```python
from build123d import *

# Parameters (mm, degrees)
SKETCH1_W             = 50.8
SKETCH1_H             = 50.8
SKETCH1_R             = 5.55625
BOSS_EXTRUDE1_DEPTH   = 1.5875
F_8_CLEARANCE_HOLE1_D = 4.3053
FILLET1_R             = 2.54


with BuildPart() as part:
    # Sketch1 → Boss-Extrude1 (new, symmetric)
    with BuildSketch(Plane.XY):
        Rectangle(SKETCH1_W, SKETCH1_H)
        Circle(SKETCH1_R, mode=Mode.SUBTRACT)
    extrude(amount=BOSS_EXTRUDE1_DEPTH, both=True)

    # #8 Clearance Hole1 (through all)
    with Locations(Plane.XY.offset(1.5875)):
        with Locations((-15.875, 15.875), (15.875, 15.875), (15.875, -15.875), (-15.875, -15.875), (0, 0)):
            Hole(F_8_CLEARANCE_HOLE1_D / 2)

    # Fillet1
    fillet1_edges = [part.edges().sort_by_distance(p)[0] for p in [
        (25.4, -25.4, 0),
        (-25.4, -25.4, 0),
        (-25.4, 25.4, 0),
        (25.4, 25.4, 0),
    ]]
    fillet(fillet1_edges, radius=FILLET1_R)


solid = part.part
```
Model file for the job. Use its own axes, mm. Coordinates: 2 decimals unless noted, no trailing zeros. Write each loop counter-clockwise with the first axis right and the second up, starting at its lowest first coordinate (ties: lowest second). Pieces come first, ordered by that corner, then holes. Notation, with made-up numbers: (9, 37.5) - (25, 37.5) arc R16 cw to (25, 66.5) - close; hole circle Ø9 at (42.5, 89.5). An arc over 180 degrees is marked (long way). One line per item, written item: value. Start each with the question number.
1. Probe line 1 (Y direction, x = 14, z = 0.15); line 2 (X direction, y = -17.5, z = 0.85); line 3 (Y direction, x = 0, z = -0.55). List the from-to ranges inside material, lowest first. Write a range as from..to.
2. Slice it at B-B (x = 2). Write the cut outline in (y, z), plus the area to 3 significant figures.
3. Mould opens along Y. For faces 1 (the cylindrical face through (-15.59, 18.01, -0.02)), 2 (the flat face through (25.4, 0, 0)), 3 (the flat face through (0, 25.4, 0)) say: released by +Y, released by -Y, zero draft, split by the parting line, or undercut.
4. Slice it at A-A (y = 0). Write the cut outline in (x, z).
5. Slice it at C-C (z = -0.85). Write the cut outline in (x, y) (1 decimal).
Answers below:
1. line 1: y = -25.4..-16.93, -14.82..14.82, 16.93..25.4
1. line 2: x = -25.4..-17.29, -14.46..14.46, 17.29..25.4
1. line 3: y = -25.4..-5.56, 5.56..25.4
2. outline: (-25.4, -1.59) - (-5.18, -1.59) - (-5.18, 1.59) - (-25.4, 1.59) - close; (5.18, -1.59) - (25.4, -1.59) - (25.4, 1.59) - (5.18, 1.59) - close
2. area: 128 mm^2
3. face 1: undercut
3. face 2: zero draft
3. face 3: released by +Y
4. outline: (-25.4, -1.59) - (-5.56, -1.59) - (-5.56, 1.59) - (-25.4, 1.59) - close; (5.56, -1.59) - (25.4, -1.59) - (25.4, 1.59) - (5.56, 1.59) - close
5. outline: (-25.4, -22.9) arc R2.5 ccw to (-22.9, -25.4) - (22.9, -25.4) arc R2.5 ccw to (25.4, -22.9) - (25.4, 22.9) arc R2.5 ccw to (22.9, 25.4) - (-22.9, 25.4) arc R2.5 ccw to (-25.4, 22.9) - close; hole circle Ø4.3 at (-15.9, -15.9); hole circle Ø4.3 at (-15.9, 15.9); hole circle Ø11.1 at (0, 0); hole circle Ø4.3 at (15.9, -15.9); hole circle Ø4.3 at (15.9, 15.9)
